Geometry check sheet. Reference: drawing and pictorial views, mm from the part's lowest x, y, z. A direction names the side the tool comes from. Coordinates: 2 decimals unless noted, no trailing zeros. Write each loop counter-clockwise with the first axis right and the second up, starting at its lowest first coordinate (ties: lowest second). Pieces come first, ordered by that corner, then holes. Notation, with made-up numbers: (19.25, -6.5) -> (76.25, -6.5) arc R13 ccw to (76.25, 8.5) -> close; hole circle Ø3 at (76, 24). An arc over 180 degrees is marked (long way). Use a Markdown table: item, result.
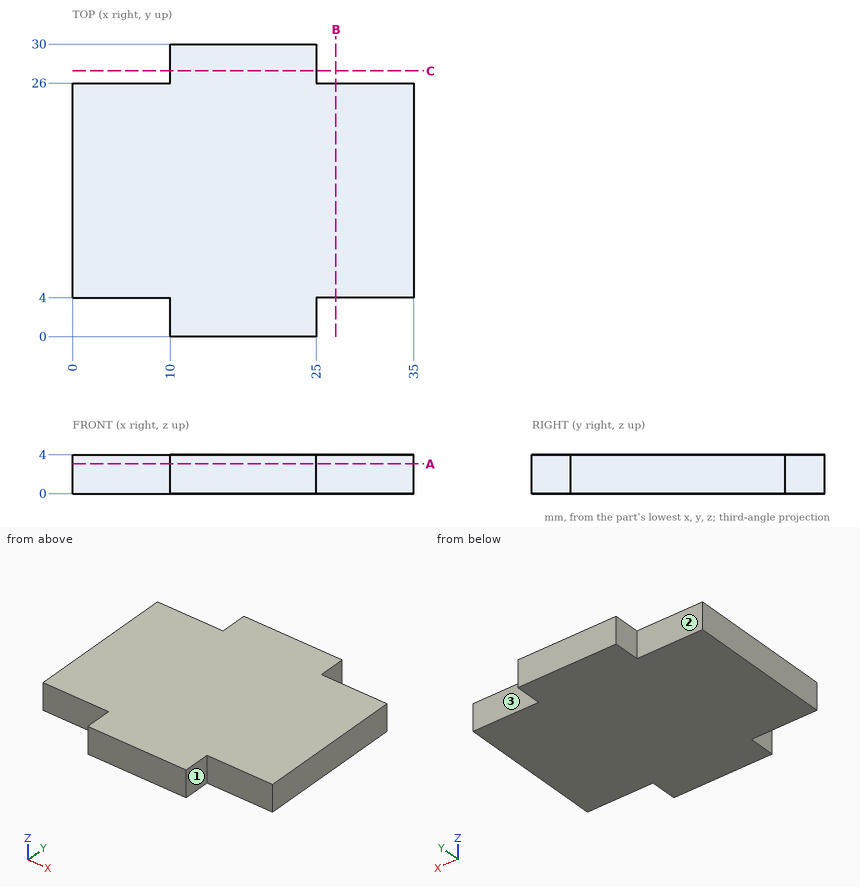
Item 1: Depth check by flat-ended pin: P1, Ø1.2, axis at x = 29, z = 2.5, coming from the +Y side; P2, Ø1.5, axis at x = 27, z = 2, coming from the -Y side; P3, Ø2, axis at y = 1.5, z = 1.5, coming from the -X side. Enter the tip coordinate at first touch or a pass-through.
Answer block:
| item | result |
|---|---|
| P1 | stops at y = 26 |
| P2 | stops at y = 4 |
| P3 | stops at x = 10 |
Item 2: Section check B-B on x = 27. Record the boundary of the cut face in (y, z), then the cut area to 3 significant figures.
Answer block:
| item | result |
|---|---|
| outline | (4, 0) -> (26, 0) -> (26, 4) -> (4, 4) -> close |
| area | 88.0 mm^2 |
Item 3: Section check A-A on z = 3.05. Record the boundary of the cut face in (x, y), then the cut area to 3 significant figures.
Answer block:
| item | result |
|---|---|
| outline | (0, 4) -> (10, 4) -> (10, 0) -> (25, 0) -> (25, 4) -> (35, 4) -> (35, 26) -> (25, 26) -> (25, 30) -> (10, 30) -> (10, 26) -> (0, 26) -> close |
| area | 890 mm^2 |
Item 4: Thickness scan on L1, parallel to Y at x = 9, z = 3.25; L2, parallel to X at y = 3.25, z = 1.85. Record the ranges inside material, lowest first. Write a range as [from, to].
Answer block:
| item | result |
|---|---|
| L1 | y = [4, 26] |
| L2 | x = [10, 25] |
Item 5: Tool access check on the marked faces 1, 2 and 3. Record the directions out of +Z, -Z, +X, -X, +Y, -Y that give a thin tool (end or side, any length) a straight path to the whole face; none if there is none.
Answer block:
| item | result |
|---|---|
| face 1 | +Z, -Z, +X, -Y |
| face 2 | +Z, -Z, -X, +Y |
| face 3 | +Z, -Z, +X, +Y |
Item 6: Section check C-C on y = 27.25. Record the boundary of the cut face in (x, z).
Answer block:
| item | result |
|---|---|
| outline | (10, 0) -> (25, 0) -> (25, 4) -> (10, 4) -> close |
